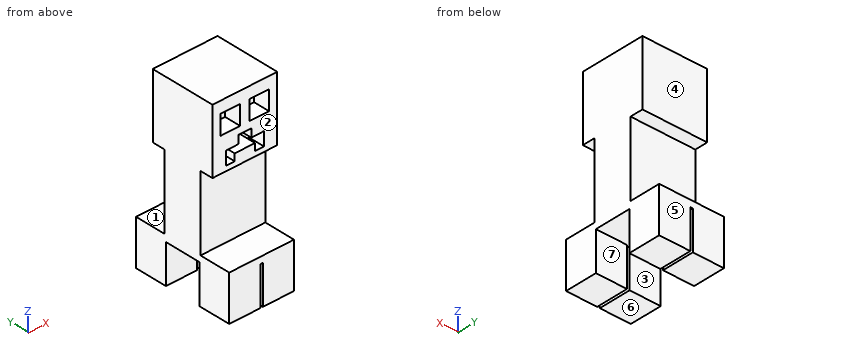
```python
from build123d import *

# Parameters (mm, degrees)
F0_W     = 100
F0_H     = 100
F1_DEPTH = 100
F2_W     = 30
F2_H     = 30
F3_DEPTH = 25
F4_W     = 50
F4_H     = 30
F5_DEPTH = 115
F6_W     = 100
F6_H     = 156
F7_DEPTH = 10
F8_W     = 48
F8_H     = 50
F9_DEPTH = 60


with BuildPart() as f1:
    # F0 (on Top) → F1 (new body)
    with BuildSketch(Plane.XY):
        Rectangle(F0_W, F0_H)
    extrude(amount=F1_DEPTH)

    # F2 (on face) → F3 (cut)
    with BuildSketch(Plane.XZ.offset(50)):
        with Locations((-22.308369, 67.011483)):
            Rectangle(F2_W, F2_H)
        with Locations((22.308369, 67.011483)):
            Rectangle(F2_W, F2_H)
        Polygon((9.954443, 40.98089), (0, 40.98089), (-9.954443, 40.98089), (-9.954443, 28.341211), (-29.406976, 28.341211), (-29.406976, 7.562513), (-15.657233, 7.562513), (-15.657233, 18.356016), (0, 18.356016), (15.657233, 18.356016), (15.657233, 7.562513), (29.406976, 7.562513), (29.406976, 28.341211), (9.954443, 28.341211), align=None)
    extrude(amount=-F3_DEPTH, mode=Mode.SUBTRACT)

    # F4 (on face) → F5 (join)
    with BuildSketch(Plane(origin=(0, 0, 0), x_dir=(1, 0, 0), z_dir=(0, 0, -1))):
        with Locations((25, -15)):
            Rectangle(F4_W, F4_H)
        with Locations((25, 15)):
            Rectangle(F4_W, F4_H)
        with Locations((-25, -15)):
            Rectangle(F4_W, F4_H)
        with Locations((-25, 15)):
            Rectangle(F4_W, F4_H)
    extrude(amount=F5_DEPTH)

    # F6 (on face) → F7 (join)
    with BuildSketch(Plane(origin=(0, 0, -115), x_dir=(1, 0, 0), z_dir=(0, 0, -1))):
        Rectangle(F6_W, F6_H)
    extrude(amount=F7_DEPTH)

    # F8 (on face) → F9 (join)
    with BuildSketch(Plane(origin=(0, 0, -125), x_dir=(1, 0, 0), z_dir=(0, 0, -1))):
        with Locations((-26, 53)):
            Rectangle(F8_W, F8_H)
        with Locations((26, 53)):
            Rectangle(F8_W, F8_H)
        with Locations((-26, -53)):
            Rectangle(F8_W, F8_H)
        with Locations((26, -53)):
            Rectangle(F8_W, F8_H)
    extrude(amount=F9_DEPTH)


solid = f1.part
```
CAD build for the part. Positions are in the model's coordinates, mm. Face numbers are marked on the shaded views. A direction names the side the tool comes from. Round coordinates to 2 decimals unless told otherwise and drop trailing zeros. Order: outer loops, then holes, each group sorted by start corner. A loop starts at its lowest first (then second) coordinate and runs counter-clockwise, first axis right, second up.
Item 1: Tool access for the marked faces 1, 2, 3 and 4: list every direction of +Z, -Z, +X, -X, +Y, -Y with a clear straight run to the whole face (end or side of a thin tool).
Item 2: Mould opens along Y. For the marked faces 5, 6 and 7 say: pulls with the +Y half, pulls with the -Y half, needs draft (parallel to the pull), parting line crosses it, or undercut.
Item 3: Saw through at D-D on z = 63. Write the cut outline in (x, y), then the cut area to 3 significant figures.
Item 4: Pin check, flat tips, straight feed: pin 1 (14.5 mm diameter, centred on x = -9.5, y = 59.5, fed in from +Z); pin 2 (8 mm diameter, centred on x = 17, y = 12, fed in from -Z); pin 3 (6 mm diameter, centred on x = -39.5, z = -68.5, fed in from +Y). Stop position of each tip, or through.
Item 5: Probe line 1 along Y through (x, z) = (-30.5, -138); line 2 along Z through (x, y) = (6.5, -40); line 3 along X through (y, z) = (70.5, -141.5). List the from-to ranges inside material, lowest first.
Item 6: Saw through at C-C on x = 24.5. Write the cut outline in (y, z), then the cut area to 3 significant figures.
Item 7: Saw through at B-B on y = 40.5. Write the cut outline in (x, z).
Item 8: Saw through at A-A on z = -158. Write the cut outline in (x, y).
Reported:
1. face 1: +X, -X, +Y
1. face 2: +Z, +X, -X, -Y
1. face 3: -Z, +X, -X
1. face 4: +Z, +X, -X, +Y
2. face 5: pulls with the +Y half
2. face 6: needs draft
2. face 7: undercut
3. outline: (-50, -50) - (-37.31, -50) - (-37.31, -25) - (-7.31, -25) - (-7.31, -50) - (7.31, -50) - (7.31, -25) - (37.31, -25) - (37.31, -50) - (50, -50) - (50, 50) - (-50, 50) - close
3. area: 8,500 mm2
4. pin 1: stops at z = -115
4. pin 2: stops at z = -125
4. pin 3: stops at y = 30
5. line 1: y = -78 to -28, 28 to 78
5. line 2: z = -185 to -115, 0 to 18.36, 40.98 to 100
5. line 3: x = -50 to -2, 2 to 50
6. outline: (-78, -185) - (-28, -185) - (-28, -125) - (28, -125) - (28, -185) - (78, -185) - (78, -115) - (30, -115) - (30, 0) - (50, 0) - (50, 100) - (-50, 100) - (-50, 82.01) - (-25, 82.01) - (-25, 52.01) - (-50, 52.01) - (-50, 28.34) - (-25, 28.34) - (-25, 7.56) - (-50, 7.56) - (-50, 0) - (-30, 0) - (-30, -115) - (-78, -115) - close
6. area: 23,200 mm2
7. outline: (-50, -185) - (-2, -185) - (-2, -125) - (2, -125) - (2, -185) - (50, -185) - (50, -115) - (-50, -115) - close; (-50, 0) - (50, 0) - (50, 100) - (-50, 100) - close
8. outline: (-50, -78) - (-2, -78) - (-2, -28) - (-50, -28) - close; (-50, 28) - (-2, 28) - (-2, 78) - (-50, 78) - close; (2, -78) - (50, -78) - (50, -28) - (2, -28) - close; (2, 28) - (50, 28) - (50, 78) - (2, 78) - close
